Input: part model. Units: mm. Frame: model coordinates. A direction names the side the tool comes from. Round coordinates to 2 decimals unless told otherwise and drop trailing zeros. Order: outer loops, then holes, each group sorted by start corner. A loop starts at its lowest first (then second) coordinate and runs counter-clockwise, first axis right, second up.
Item 1: Line query: L1, parallel to X at y = 9.2, z = -33.5; L2, parallel to X at y = 7.5, z = -6. Output: solid intervals per line, ascending.
Item 2: Cut plane C-C on z = -64. Output: boundary loops of the cut face in (x, y), then the cut area to 3 significant figures.
Item 3: Reachability of faces 1 (the flat face through (-10, 0, 2)), 2 (the flat face through (8.5, 0, 2)) from +Z, -Z, +X, -X, +Y, -Y: full face, straight path, thin tool, end or side. Return the list, or none.
Item 4: First-contact query: pin 1 (3 mm diameter, centred on x = -6, z = -33.5, fed in from +Y). Flat tip, straight axial feed; report the tip coordinate or a pass-through.
Item 5: Mould query, pull axis Z, two halves, no side actions, for faces 3 (the cylindrical face through (-9.24, -0.56, 7.46)), 4 (the cylindrical face through (-9.24, -0.56, -57.54)), 5 (the flat face through (0, 10, 2)), 6 (the flat face through (-9, 0, -112.5)). Classes: released by +Z, released by -Z, zero draft, split by the parting line, or undercut.
Item 6: Cut plane A-A on z = 30. Output: boundary loops of the cut face in (x, y), then the cut area to 3 significant figures.
Item 7: Cut plane B-B on y = 4.75. Output: boundary loops of the cut face in (x, z).
```python
from build123d import *

# Parameters (mm, degrees)
SKETCH_1_W          = 20
SKETCH_1_H          = 20
SKETCH_1_W_2        = 17
SKETCH_1_H_2        = 17
EXTRUDE_1_DEPTH     = 112.5
SKETCH_2_R          = 2.55
CUT_EXTRUDE_1_DEPTH = 115.70069747
SKETCH_3_R          = 2.6
CUT_EXTRUDE_2_DEPTH = 115.70069747
SKETCH_4_R          = 1.55
CUT_EXTRUDE_3_DEPTH = 115.70069747


with BuildPart() as part:
    # 草图1 → 凸台-拉伸1 (new, symmetric)
    with BuildSketch(Plane.XY):
        Rectangle(SKETCH_1_W, SKETCH_1_H)
        Rectangle(SKETCH_1_W_2, SKETCH_1_H_2, mode=Mode.SUBTRACT)
    extrude(amount=EXTRUDE_1_DEPTH, both=True)

    # 草图2 → 切除-拉伸1 (cut, through all)
    with BuildSketch(Plane(origin=(0, 10, 0), x_dir=(1, 0, 0), z_dir=(0, 1, 0))):
        with Locations(Location((0, -72.5, 0), (0, 0, 270))):
            Circle(SKETCH_2_R)
        with Locations(Location((0, -44.5, 0), (0, 0, 270))):
            Circle(SKETCH_2_R)
    extrude(amount=-CUT_EXTRUDE_1_DEPTH, mode=Mode.SUBTRACT)

    # 草图3 → 切除-拉伸2 (cut, through all)
    with BuildSketch(Plane(origin=(10, 0, 0), x_dir=(0, 0, -1), z_dir=(1, 0, 0))):
        with Locations(Location((85, 0, 0), (0, 0, 90))):
            Circle(SKETCH_3_R)
        with Locations(Location((55, 0, 0), (0, 0, 90))):
            Circle(SKETCH_3_R)
        with Locations(Location((35, 0, 0), (0, 0, 90))):
            Circle(SKETCH_3_R)
        with Locations(Location((-10, 0, 0), (0, 0, 90))):
            Circle(SKETCH_3_R)
        with Locations(Location((-20, 0, 0), (0, 0, 90))):
            Circle(SKETCH_3_R)
        with Locations(Location((-30, 0, 0), (0, 0, 90))):
            Circle(SKETCH_3_R)
        with Locations(Location((-75, 0, 0), (0, 0, 90))):
            Circle(SKETCH_3_R)
        with Locations(Location((-95, 0, 0), (0, 0, 90))):
            Circle(SKETCH_3_R)
    extrude(amount=-CUT_EXTRUDE_2_DEPTH, mode=Mode.SUBTRACT)

    # 草图4 → 切除-拉伸3 (cut, through all)
    with BuildSketch(Plane(origin=(0, 10, 0), x_dir=(1, 0, 0), z_dir=(0, 1, 0))):
        with Locations(Location((-6, 3.5, 0), (0, 0, 270))):
            Circle(SKETCH_4_R)
        with Locations(Location((6, 3.5, 0), (0, 0, 270))):
            Circle(SKETCH_4_R)
        with Locations(Location((-6, 33.5, 0), (0, 0, 270))):
            Circle(SKETCH_4_R)
        with Locations(Location((6, 33.5, 0), (0, 0, 270))):
            Circle(SKETCH_4_R)
    extrude(amount=-CUT_EXTRUDE_3_DEPTH, mode=Mode.SUBTRACT)


solid = part.part
```
From the geometry:
1. L1: x = -10 to -7.55, -4.45 to 4.45, 7.55 to 10
1. L2: x = -10 to -8.5, 8.5 to 10
2. outline: (-10, -10) - (10, -10) - (10, 10) - (-10, 10) - close; hole (-8.5, -8.5) - (8.5, -8.5) - (8.5, 8.5) - (-8.5, 8.5) - close
2. area: 111 mm2
3. face 1: +Z, -Z, -X, +Y, -Y
3. face 2: +Z, -Z
4. pin 1: passes through
5. face 3: undercut
5. face 4: undercut
5. face 5: zero draft
5. face 6: released by -Z
6. outline: (-10, -10) - (10, -10) - (10, -2.6) - (8.5, -2.6) - (8.5, -8.5) - (-8.5, -8.5) - (-8.5, -2.6) - (-10, -2.6) - close; (-10, 2.6) - (-8.5, 2.6) - (-8.5, 8.5) - (8.5, 8.5) - (8.5, 2.6) - (10, 2.6) - (10, 10) - (-10, 10) - close
6. area: 95.4 mm2
7. outline: (-10, -112.5) - (-8.5, -112.5) - (-8.5, 112.5) - (-10, 112.5) - close; (8.5, -112.5) - (10, -112.5) - (10, 112.5) - (8.5, 112.5) - close
